Build history of the part. All positions in model axes, mm. Face numbers are marked on the shaded views. Round coordinates to 2 decimals unless told otherwise and drop trailing zeros. Write each loop counter-clockwise with the first axis right and the second up, starting at its lowest first coordinate (ties: lowest second). Pieces come first, ordered by that corner, then holes. Notation, with made-up numbers: (9, 6) -> (20, 6) arc R21 ccw to (20, 16) -> close; hole circle Ø11 at (10.5, 38.25). An arc over 180 degrees is marked (long way). Return JSON: item names as keys, results as strings.
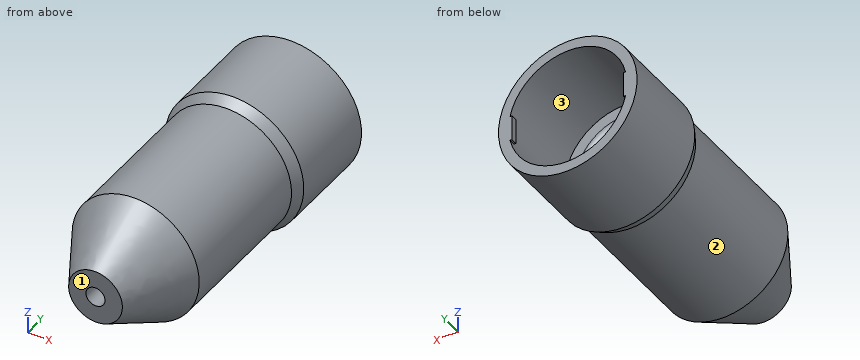
from build123d import *

# Parameters (mm, degrees)
SKETCH1_R           = 5
SKETCH1_R_2         = 2.75
BOSS_EXTRUDE1_DEPTH = 16
BOSS_EXTRUDE2_START = 1.5
SKETCH2_R           = 5
BOSS_EXTRUDE2_DEPTH = 1.5
SKETCH3_R           = 0.75
CUT_EXTRUDE1_DEPTH  = 1.5
CHAMFER1_SIZE       = 5
CHAMFER1_SIZE2      = 2.886751346
CHAMFER2_SIZE       = 2
CHAMFER2_SIZE2      = 1.154700538
FILLET1_R           = 1
SKETCH5_R           = 5.45
SKETCH5_R_2         = 4.65
BOSS_EXTRUDE4_DEPTH = 7
CHAMFER4_SIZE       = 0.554309051
CHAMFER4_SIZE_2     = 1
SKETCH6_W           = 0.5
SKETCH6_H           = 2
BOSS_EXTRUDE5_DEPTH = 0.5


with BuildPart() as part:
    # Sketch1 → Boss-Extrude1 (new body)
    with BuildSketch(Plane(origin=(0, 0, 0), x_dir=(1, 0, 0), z_dir=(0, 1, 0))):
        with Locations(Location((0, 0, 0), (0, 0, 270))):
            Circle(SKETCH1_R)
        with Locations(Location((0, 0, 0), (0, 0, 270))):
            Circle(SKETCH1_R_2, mode=Mode.SUBTRACT)
    extrude(amount=BOSS_EXTRUDE1_DEPTH)

    # Sketch2 → Boss-Extrude2 (add)
    with BuildSketch(Plane.XZ.offset(BOSS_EXTRUDE2_START)):
        with Locations(Location((0, 0, 0), (0, 0, 270))):
            Circle(SKETCH2_R)
    extrude(amount=-BOSS_EXTRUDE2_DEPTH)

    # Sketch3 → Cut-Extrude1 (cut)
    with BuildSketch(Plane(origin=(0, 0, 0), x_dir=(1, 0, 0), z_dir=(0, 1, 0))):
        with Locations(Location((0, 0, 0), (0, 0, 270))):
            Circle(SKETCH3_R)
    extrude(amount=-CUT_EXTRUDE1_DEPTH, mode=Mode.SUBTRACT)

    # Chamfer1
    chamfer1_edges = [part.edges().sort_by_distance(p)[0] for p in [
        (0, -1.5, 5),
    ]]
    chamfer1_side = [part.faces().sort_by_distance(p)[0] for p in [
        (0, -0.75, 5),
    ]]
    chamfer(chamfer1_edges, length=CHAMFER1_SIZE, length2=CHAMFER1_SIZE2, reference=chamfer1_side[0])

    # Chamfer2
    chamfer2_edges = [part.edges().sort_by_distance(p)[0] for p in [
        (0, 0, -2.75),
    ]]
    chamfer2_side = [part.faces().sort_by_distance(p)[0] for p in [
        (0, 8, -2.75),
    ]]
    chamfer(chamfer2_edges, length=CHAMFER2_SIZE, length2=CHAMFER2_SIZE2, reference=chamfer2_side[0])

    # Fillet1
    fillet1_edges = [part.edges().sort_by_distance(p)[0] for p in [
        (0, 16, -2.75),
    ]]
    fillet(fillet1_edges, radius=FILLET1_R)

    # Sketch5 → Boss-Extrude4 (add)
    with BuildSketch(Plane(origin=(0, 16, 0), x_dir=(1, 0, 0), z_dir=(0, 1, 0))):
        with Locations(Location((0, 0, 0), (0, 0, 270))):
            Circle(SKETCH5_R)
        with Locations(Location((0, 0, 0), (0, 0, 270))):
            Circle(SKETCH5_R_2, mode=Mode.SUBTRACT)
    extrude(amount=BOSS_EXTRUDE4_DEPTH)

    # Chamfer4
    # the kernel refuses this chamfer: 1, 0.554309051 mm, written as the material it adds along each edge
    with BuildSketch(Plane(origin=(0, 16, 0), x_dir=(0, 0, 1), z_dir=(-1, 0, 0))) as chamfer4_piece_1_section:
        Polygon((5 + CHAMFER4_SIZE, 0), (5, -CHAMFER4_SIZE_2), (5, 0), align=None)
    chamfer4_piece_1 = revolve(axis=Axis((0, 16, 0), (0, 1, 0)), mode=Mode.PRIVATE)
    chamfer4_piece_1 = chamfer4_piece_1 & Plane(origin=(0, 15.398774121, 0), x_dir=(0, 0, 1), z_dir=(0, -1, 0)) * Cylinder(5.45, 23, mode=Mode.PRIVATE)
    add(chamfer4_piece_1)

    # Sketch6 → Boss-Extrude5 (add)
    with BuildSketch(Plane(origin=(0, 23, 0), x_dir=(1, 0, 0), z_dir=(0, 1, 0))):
        with Locations((4.65, 0)):
            Rectangle(SKETCH6_W, SKETCH6_H)
        with Locations((-4.65, 0)):
            Rectangle(SKETCH6_W, SKETCH6_H)
    extrude(amount=-BOSS_EXTRUDE5_DEPTH)


solid = part.part
Q1. Pin check, flat tips, straight feed: pin 1 Ø2.5 at (x, z) = (0.5, -0.5) entering from +Y; pin 2 Ø5 at (y, z) = (15, -0.5) entering from -X; pin 3 Ø5 at (y, z) = (16.5, -4) entering from +X; pin 4 Ø1.5 at (x, y) = (-3.5, 13.5) entering from +Z. Stop position of each tip, or through.
Verdict:
{"pin 1": "stops at y = 0.63", "pin 2": "stops at x = -5.45", "pin 3": "stops at x = 5.24", "pin 4": "stops at z = 4.18"}
Q2. Two-plate mould, pull along Z, no slides. Class the marked faces 1, 2 and 3: +Z half, -Z half, draft (parallel to the pull), parting line (faces both ways), or undercut.
Verdict:
{"face 1": "draft", "face 2": "parting line", "face 3": "undercut"}
Q3. Saw through at A-A on y = 6. List the corners of the cut face in (x, z), then the cut area to 3 significant figures.
Verdict:
{"outline": "circle Ø10 at (0, 0); hole circle Ø5.5 at (0, 0)", "area": "54.8 mm²"}
Q4. Wall check: L1, parallel to X at y = 11.5, z = 0; L2, parallel to X at y = 17.5, z = 0; L3, parallel to Z at x = -2.25, y = 2.5. Give the ranges that are in metal, low to high.
Verdict:
{"L1": "x = -5 to -2.75, 2.75 to 5", "L2": "x = -5.45 to -4.65, 4.65 to 5.45", "L3": "z = -3.81 to -1.58, 1.58 to 3.81"}
